```python
from build123d import *

# Parameters (mm, degrees)
MAINBODYS_R           = 2.5
MAIN_BODY_DEPTH       = 2
M3X0_5_TAPPED_HOLE1_D = 2.5
GROOVED_CUT_DEPTH     = 6.338539126
GC_START              = -2
GC_CP_DEPTH           = 4
PRESSFITBODYS_R       = 2
PRESSFITBODYS_R_2     = 1.25
PRESS_FIT_BODY_DEPTH  = 2.5


# Read off the part's stored shape, not the designer's step: GC CP
with BuildPart() as part:
    # MainBodyS → MAIN BODY (new, symmetric)
    with BuildSketch(Plane(origin=(0, 0, 0), x_dir=(1, 0, 0), z_dir=(0, 1, 0))):
        with Locations(Location((0, 0, 0), (0, 0, 270))):
            Circle(MAINBODYS_R)
    extrude(amount=MAIN_BODY_DEPTH, both=True)

    # M3x0.5 Tapped Hole1 (through all)
    with Locations(Plane(origin=(0, 2, 0), x_dir=(1, 0, 0), z_dir=(0, 1, 0))):
        with Locations((0, 0)):
            Hole(M3X0_5_TAPPED_HOLE1_D / 2)

    # GroovedCutS → GROOVED CUT (cut, through all)
    with BuildSketch(Plane(origin=(0, 2, 0), x_dir=(1, 0, 0), z_dir=(0, 1, 0))):
        with BuildLine():
            Line((0, 2.25), (0.382129822, 2.470622755))
            ThreePointArc((0.382129822, 2.470622755), (0, 2.5), (-0.382129822, 2.470622755))
            Line((-0.382129822, 2.470622755), (0, 2.25))
        make_face()
    extrude(amount=-GROOVED_CUT_DEPTH, mode=Mode.SUBTRACT)

    # GC CP outline → GC CP (cut)
    with BuildSketch(Plane(origin=(0, 0, 0), x_dir=(1, 0, 0), z_dir=(0, 1, 0)).offset(GC_START)):
        with BuildLine():
            ThreePointArc((-0.727675966, 2.391754103), (-1.084709348, 2.25242217), (-1.416250112, 2.060154271))
            Line((-1.416250112, 2.060154271), (-0.976238413, 2.027179953))
            Line((-0.976238413, 2.027179953), (-0.727675966, 2.391754103))
        make_face()
        with BuildLine():
            Line((0.976238413, 2.027179953), (1.416250112, 2.060154271))
            ThreePointArc((1.416250112, 2.060154271), (1.084709348, 2.25242217), (0.727675966, 2.391754103))
            Line((0.727675966, 2.391754103), (0.976238413, 2.027179953))
        make_face()
        with BuildLine():
            Line((1.759120836, 1.402852054), (2.169864698, 1.241646967))
            ThreePointArc((2.169864698, 1.241646967), (1.954578706, 1.558724504), (1.693356605, 1.839169217))
            Line((1.693356605, 1.839169217), (1.759120836, 1.402852054))
        make_face()
        with BuildLine():
            Line((2.193587802, 0.500672101), (2.493710969, 0.177216254))
            ThreePointArc((2.493710969, 0.177216254), (2.43731978, 0.556302335), (2.3236472, 0.922314312))
            Line((2.3236472, 0.922314312), (2.193587802, 0.500672101))
        make_face()
        with BuildLine():
            Line((2.193587802, -0.500672101), (2.3236472, -0.922314312))
            ThreePointArc((2.3236472, -0.922314312), (2.43731978, -0.556302335), (2.493710969, -0.177216254))
            Line((2.493710969, -0.177216254), (2.193587802, -0.500672101))
        make_face()
        with BuildLine():
            Line((1.759120836, -1.402852054), (1.693356605, -1.839169217))
            ThreePointArc((1.693356605, -1.839169217), (1.954578706, -1.558724504), (2.169864698, -1.241646967))
            Line((2.169864698, -1.241646967), (1.759120836, -1.402852054))
        make_face()
        with BuildLine():
            Line((0.976238413, -2.027179953), (0.727675966, -2.391754103))
            ThreePointArc((0.727675966, -2.391754103), (1.084709348, -2.25242217), (1.416250112, -2.060154271))
            Line((1.416250112, -2.060154271), (0.976238413, -2.027179953))
        make_face()
        with BuildLine():
            Line((0, -2.25), (-0.382129822, -2.470622755))
            ThreePointArc((-0.382129822, -2.470622755), (0, -2.5), (0.382129822, -2.470622755))
            Line((0.382129822, -2.470622755), (0, -2.25))
        make_face()
        with BuildLine():
            Line((-0.976238413, -2.027179953), (-1.416250112, -2.060154271))
            ThreePointArc((-1.416250112, -2.060154271), (-1.084709348, -2.25242217), (-0.727675966, -2.391754103))
            Line((-0.727675966, -2.391754103), (-0.976238413, -2.027179953))
        make_face()
        with BuildLine():
            Line((-1.759120836, -1.402852054), (-2.169864698, -1.241646967))
            ThreePointArc((-2.169864698, -1.241646967), (-1.954578706, -1.558724504), (-1.693356605, -1.839169217))
            Line((-1.693356605, -1.839169217), (-1.759120836, -1.402852054))
        make_face()
        with BuildLine():
            Line((-2.193587802, -0.500672101), (-2.493710969, -0.177216254))
            ThreePointArc((-2.493710969, -0.177216254), (-2.43731978, -0.556302335), (-2.3236472, -0.922314312))
            Line((-2.3236472, -0.922314312), (-2.193587802, -0.500672101))
        make_face()
        with BuildLine():
            Line((-2.193587802, 0.500672101), (-2.3236472, 0.922314312))
            ThreePointArc((-2.3236472, 0.922314312), (-2.43731978, 0.556302335), (-2.493710969, 0.177216254))
            Line((-2.493710969, 0.177216254), (-2.193587802, 0.500672101))
        make_face()
        with BuildLine():
            Line((-1.759120836, 1.402852054), (-1.693356605, 1.839169217))
            ThreePointArc((-1.693356605, 1.839169217), (-1.954578706, 1.558724504), (-2.169864698, 1.241646967))
            Line((-2.169864698, 1.241646967), (-1.759120836, 1.402852054))
        make_face()
    extrude(amount=GC_CP_DEPTH, mode=Mode.SUBTRACT)

    # PressFitBodyS → PRESS FIT BODY (add)
    with BuildSketch(Plane(origin=(0, 2, 0), x_dir=(1, 0, 0), z_dir=(0, 1, 0))):
        with Locations(Location((0, 0, 0), (0, 0, 270))):
            Circle(PRESSFITBODYS_R)
        with Locations(Location((0, 0, 0), (0, 0, 270))):
            Circle(PRESSFITBODYS_R_2, mode=Mode.SUBTRACT)
    extrude(amount=PRESS_FIT_BODY_DEPTH)


solid = part.part
```
Work out the finished part from the listing and answer in its coordinate system (mm). A direction names the side the tool comes from. Round coordinates to 2 decimals unless told otherwise and drop trailing zeros. Write each loop counter-clockwise with the first axis right and the second up, starting at its lowest first coordinate (ties: lowest second). Pieces come first, ordered by that corner, then holes. Notation, with made-up numbers: (-12.5, 46.5) -> (35.5, 46.5) arc R25 cw to (35.5, 81.5) -> close; hole circle Ø4 at (-12, -22). An arc over 180 degrees is marked (long way). Write each question's results on one line, items separated by ' | '.
1) The part is cut by section D-D (z = -1.6). Write down the section's boundary in (x, y).
Findings:
outline: (-1.73, -2) -> (1.73, -2) -> (1.73, 2) -> (1.2, 2) -> (1.2, 4.5) -> (-1.2, 4.5) -> (-1.2, 2) -> (-1.73, 2) -> close
2) Consider line 1 along X through (y, z) = (2.6, 0); line 2 along Y through (x, z) = (1.2, -1.7); line 3 along Z through (x, y) = (-0.05, 0.75). Determine where each line is inside the solid, lowest interval first. Write a range as [from, to].
Findings:
line 1: x = [-2, -1.25], [1.25, 2] | line 2: y = [-2, 2] | line 3: z = [-2.28, -1.25], [1.25, 2.28]
3) The part is cut by section B-B (x = 0.3). Write down the section's boundary in (y, z), and give its area (3 significant figures).
Findings:
outline: (-2, -2.42) -> (2, -2.42) -> (2, -1.98) -> (4.5, -1.98) -> (4.5, -1.21) -> (-2, -1.21) -> close; (-2, 1.21) -> (4.5, 1.21) -> (4.5, 1.98) -> (2, 1.98) -> (2, 2.42) -> (-2, 2.42) -> close | area: 13.5 mm²
4) The part is cut by section A-A (z = 0). Write down the section's boundary in (x, y).
Findings:
outline: (-2.5, -2) -> (-1.25, -2) -> (-1.25, 4.5) -> (-2, 4.5) -> (-2, 2) -> (-2.5, 2) -> close; (1.25, -2) -> (2.5, -2) -> (2.5, 2) -> (2, 2) -> (2, 4.5) -> (1.25, 4.5) -> close
5) Which of the six approach directions +Z, -Z, +X, -X, +Y, -Y give full straight-line access (tool end or side, diameter ignored) to faces 1 (the flat face through (2, 2, -1)), 2 (the flat face through (1, -2, -1))?
Findings:
face 1: +Y | face 2: +Z, -Z, +X, -X, -Y
6) A flat-ended cylindrical pin translates along its axis: pin 1 (2 mm diameter, centred on y = 1, z = -2, fed in from +X). Find the tip coordinate at first contact, or state that the pin passes through.
Findings:
pin 1: stops at x = 2.29
7) The part is cut by section C-C (y = 4.25). Write down the section's boundary in (x, z), and give its area (3 significant figures).
Findings:
outline: circle Ø4 at (0, 0); hole circle Ø2.5 at (0, 0) | area: 7.66 mm²
